For this review, use the dimensioned drawing (mm, ordinates from the lowest corner) and the shaded views. A direction names the side the tool comes from. Round coordinates to 2 decimals unless told otherwise and drop trailing zeros. Order: outer loops, then holes, each group sorted by start corner. A loop starts at its lowest first (then second) coordinate and runs counter-clockwise, first axis right, second up. Notation, with made-up numbers: M 85,-2.75 L 134,-2.75 A27 cw 134,35.25 Z; hole C -8.75,-34.5 d1. An arc over 180 degrees is marked long. Use a Markdown table: item, result. Add a question column.
1. To check wall thickness, follow probe 1 along Y at (x, z) = (152.4, 82.5); probe 2 along X at (y, z) = (175, 148) (1 decimal); probe 3 along Z at (x, y) = (95, 52). State the ranges of each line that lie inside material, in increasing order.
2. Consider section D-D on z = 143. State the section outline as (x, y) points (1 decimal), then the cut area to 3 significant figures.
3. Insertion check: P1, Ø10, axis at x = 206, z = 108.5, coming from the -Y side; P2, Ø2, axis at x = 131, z = 105, coming from the -Y side; P3, Ø8, axis at y = 261, z = 90, coming from the +X side; P4, Ø10, axis at x = 177, z = 93, coming from the +Y side. Each pin has a flat end and moves straight along its axis. Give the tip position at first contact, or say it passes through.
4. For the marked faces 4 and 5, list the 3-axis set-ups (+Z, -Z, +X, -X, +Y, -Y) from which the entire face can be reached by the end or side of a thin tool; tool diameter is ignored.
5. Consider section C-C on z = 105.5. State the section outline as (x, y) points, then the cut area to 3 significant figures.
6. Consider section A-A on x = 152.4. State the section outline as (y, z) points, then the cut area to 3 significant figures.
7. The part is to be moulded in two halves that separate along X. For the marked faces 1, 2 and 3, say which applies: +X half, -X half, draft (parallel to the pull), parting line (faces both ways), or undercut.
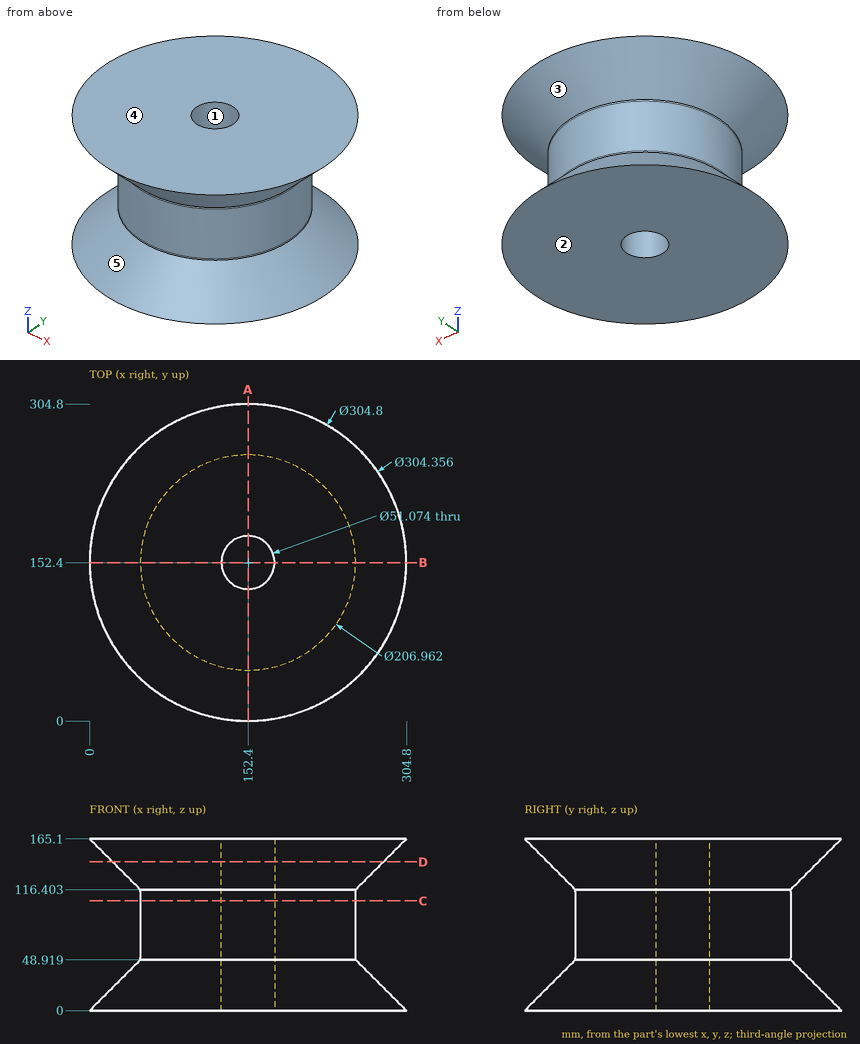
Answer block:
| question | item | result |
|---|---|---|
| 1 | probe 1 | 48.92 to 126.86, 177.94 to 255.88 |
| 1 | probe 2 | 19.2 to 140.5, 164.3 to 285.6 |
| 1 | probe 3 | 0 to 36.75, 128.57 to 165.1 |
| 2 | outline | C 152.4,152.4 d260.2; hole C 152.4,152.4 d51.1 |
| 2 | area | 51,100 mm^2 |
| 3 | P1 | y = 61.04 |
| 3 | P2 | y = 50.95 |
| 3 | P3 | through |
| 3 | P4 | y = 254.01 |
| 4 | face 4 | +Z, +X, -X, +Y, -Y |
| 4 | face 5 | none |
| 5 | outline | C 152.4,152.4 d206.96; hole C 152.4,152.4 d51.07 |
| 5 | area | 31,600 mm^2 |
| 6 | outline | M 0,0 L 126.86,0 L 126.86,165.1 L 0.22,165.1 L 48.92,116.4 L 48.92,48.92 Z; M 177.94,0 L 304.8,0 L 255.88,48.92 L 255.88,116.4 L 304.58,165.1 L 177.94,165.1 Z |
| 6 | area | 30,500 mm^2 |
| 7 | face 1 | undercut |
| 7 | face 2 | draft |
| 7 | face 3 | parting line |
